Answer from the drawing. Dimensions are ordinates in mm from the lowest x, y and z of the part. Coordinates: 2 decimals unless noted, no trailing zeros. Write each loop counter-clockwise with the first axis right and the second up, starting at its lowest first coordinate (ties: lowest second). Pieces come first, ordered by that corner, then holes.
(1) Given pin 1 (3 mm diameter, centred on x = 1.5, y = 30.5, fed in from -Z); pin 2 (1.5 mm diameter, centred on x = 7, y = 5.5, fed in from -Z), each flat-ended and moving along its own axis, determine where each tip first touches the part or whether it passes through.
(2) The part is cut by section D-D, the plane y = 36.5. Determine the outline of the cut face in (x, z), and give its area (3 significant figures).
(3) The part is cut by section C-C, the plane y = 8. Determine the outline of the cut face in (x, z), and give its area (3 significant figures).
(4) The part is cut by section B-B, the plane x = 6.5. Determine the outline of the cut face in (y, z), and give its area (3 significant figures).
(5) Straight lines are drawn through the part: line 1 along Z through (x, y) = (8.5, 20); line 2 along Y through (x, z) = (3.5, 68); line 3 along Z through (x, y) = (12.75, 13.5). For each, find the intervals that lie inside material, in ascending order.
(6) The part is cut by section A-A, the plane y = 20. Determine the outline of the cut face in (x, z), and give its area (3 significant figures).
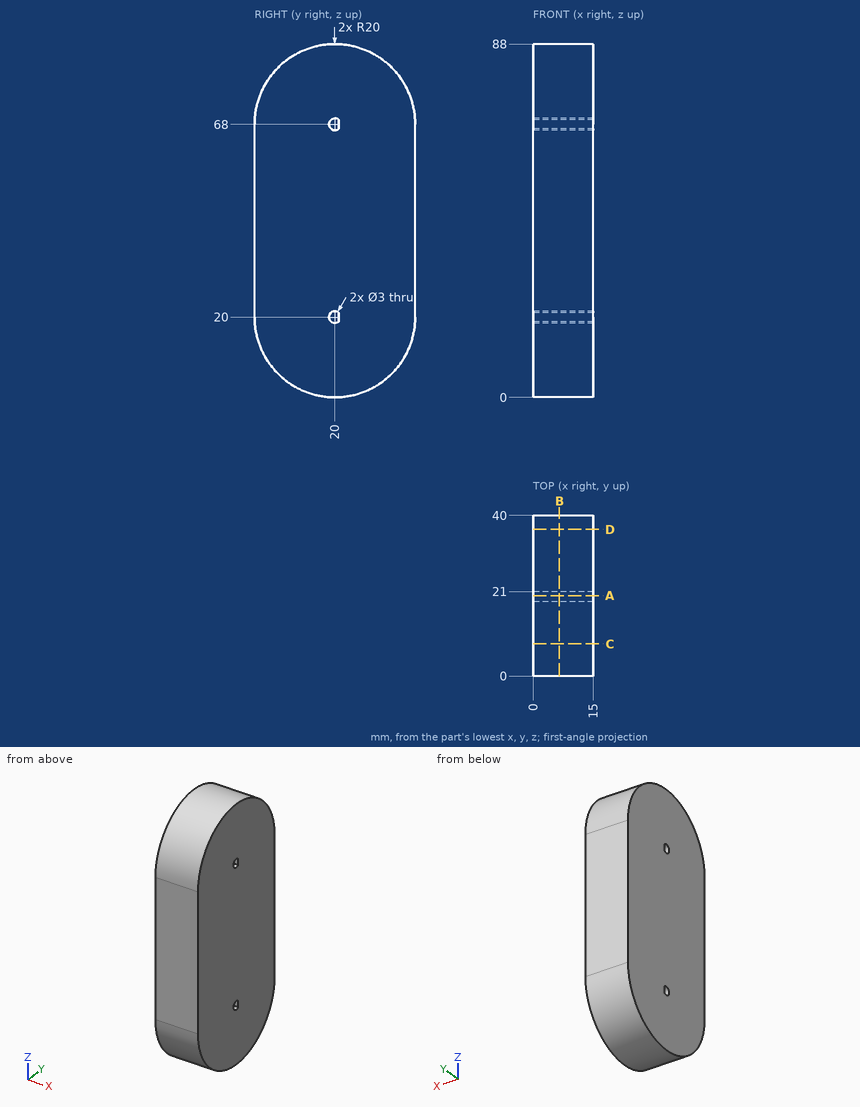
Computed:
1. pin 1: stops at z = 2.14
1. pin 2: stops at z = 5.48
2. outline: (0, 8.7) - (15, 8.7) - (15, 79.3) - (0, 79.3) - close
2. area: 1,060 mm2
3. outline: (0, 4) - (15, 4) - (15, 84) - (0, 84) - close
3. area: 1,200 mm2
4. outline: (0, 20) arc R20 ccw to (40, 20) - (40, 68) arc R20 ccw to (0, 68) - close; hole (21, 18.88) - (21, 21.12) arc R1.5 ccw (long way) to start; hole (21, 66.88) - (21, 69.12) arc R1.5 ccw (long way) to start
4. area: 3,160 mm2
5. line 1: z = 0 to 18.5, 21.5 to 66.5, 69.5 to 88
5. line 2: y = 0 to 18.5, 21 to 40
5. line 3: z = 1.09 to 86.91
6. outline: (0, 0) - (15, 0) - (15, 18.5) - (0, 18.5) - close; (0, 21.5) - (15, 21.5) - (15, 66.5) - (0, 66.5) - close; (0, 69.5) - (15, 69.5) - (15, 88) - (0, 88) - close
6. area: 1,230 mm2
